Geometry check sheet. Reference: the model listing, model coordinates, mm. Face numbers are marked on the shaded views. Round coordinates to 2 decimals unless told otherwise and drop trailing zeros. Order: outer loops, then holes, each group sorted by start corner. A loop starts at its lowest first (then second) coordinate and runs counter-clockwise, first axis right, second up. Notation, with made-up numbers: (56.25, 36.5) -> (69.25, 36.5) arc R6 ccw to (69.25, 41.5) -> close; hole circle Ø11 at (61, 24.5). An arc over 180 degrees is marked (long way). Answer as a JSON object with one key per item and string values. Group by question number.
from build123d import *

# Parameters (mm, degrees)
F1_DEPTH = 361


with BuildPart() as f1:
    # F0 (on Right) → F1 (new body, symmetric)
    with BuildSketch(Plane.YZ):
        with BuildLine():
            Line((50, 0), (0, 0))
            Line((0, 0), (0, -10))
            Line((0, -10), (45, -10))
            ThreePointArc((45, -10), (48.535534, -11.464466), (50, -15))
            Line((50, -15), (50, -97))
            ThreePointArc((50, -97), (48.535534, -100.535534), (45, -102))
            Line((45, -102), (0, -102))
            Line((0, -102), (0, -112))
            Line((0, -112), (50, -112))
            ThreePointArc((50, -112), (57.071068, -109.071068), (60, -102))
            Line((60, -102), (60, -10))
            ThreePointArc((60, -10), (57.071068, -2.928932), (50, 0))
        make_face()
    extrude(amount=F1_DEPTH, both=True)


solid = f1.part
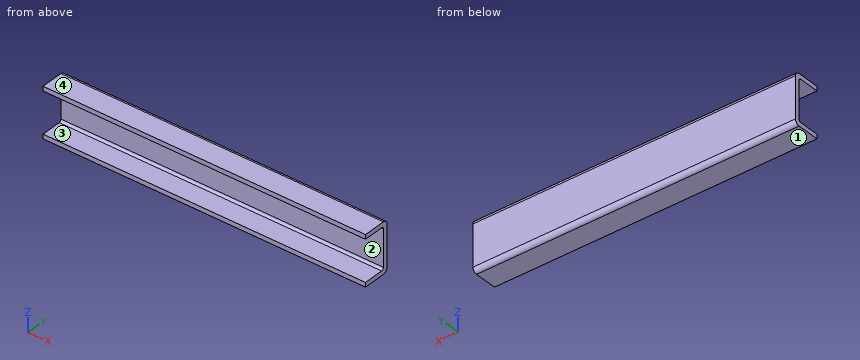
Item 1: Sectioned sample at C-C, the plane z = -44. Enter the section's corners in (x, y).
Item 2: Mould release check, pull along Z, two halves, no side actions. Record for the marked faces 1, 2, 3 and 4: pulls with the +Z half, pulls with the -Z half, needs draft (parallel to the pull), parting line crosses it, or undercut.
Item 3: Thickness scan on L1, parallel to Z at x = -148, y = 18; L2, parallel to Y at x = -239, z = -15; L3, parallel to Z at x = 160.5, y = 55. Record the ranges inside material, lowest first.
Item 4: Sectioned sample at A-A, the plane y = 8.5. Enter the section's corners in (x, z), then the cut area to 3 significant figures.
Item 5: Depth check by flat-ended pin: pin 1 Ø6 at (x, z) = (-107.5, -69) entering from -Y. Enter the tip coordinate at first touch or a pass-through.
Item 6: Sectioned sample at B-B, the plane x = -240. Enter the section's corners in (y, z).
Result:
{
 "1": {"outline": "(-361, 50) -> (361, 50) -> (361, 60) -> (-361, 60) -> close"},
 "2": {"face 1": "pulls with the -Z half", "face 2": "undercut", "face 3": "undercut", "face 4": "pulls with the +Z half"},
 "3": {"L1": "z = -112 to -102, -10 to 0", "L2": "y = 50 to 60", "L3": "z = -110.66 to -1.34"},
 "4": {"outline": "(-361, -112) -> (361, -112) -> (361, -102) -> (-361, -102) -> close; (-361, -10) -> (361, -10) -> (361, 0) -> (-361, 0) -> close", "area": "14,400 mm2"},
 "5": {"pin 1": "stops at y = 50"},
 "6": {"outline": "(0, -112) -> (50, -112) arc R10 ccw to (60, -102) -> (60, -10) arc R10 ccw to (50, 0) -> (0, 0) -> (0, -10) -> (45, -10) arc R5 cw to (50, -15) -> (50, -97) arc R5 cw to (45, -102) -> (0, -102) -> close"}
}
